Geometry check sheet. Reference: the model listing, model coordinates, mm. A direction names the side the tool comes from. Round coordinates to 2 decimals unless told otherwise and drop trailing zeros. Loops run counter-clockwise (first coordinate to the right, second up) from the corner with the lowest first, then second, coordinate; pieces in that order, holes last. Notation, with made-up numbers: (-28, 75.25) -> (21, 75.25) arc R13 ccw to (21, 85.25) -> close; hole circle Ø11 at (-36.5, -21). An arc over 180 degrees is marked (long way). Use one line per item in the form item = value.
from build123d import *

# Parameters (mm, degrees)
SKETCH1_W           = 34.925
SKETCH1_H           = 34.925
SKETCH1_R           = 1.5
BOSS_EXTRUDE1_DEPTH = 4
CUT_EXTRUDE1_DEPTH  = 5.08
FILLET1_R           = 3
CUT_EXTRUDE2_DEPTH  = 5.08


with BuildPart() as part:
    # Sketch1 → Boss-Extrude1 (new body)
    with BuildSketch(Plane.XY):
        Rectangle(SKETCH1_W, SKETCH1_H)
        with Locations((-12.7, 12.7)):
            Circle(SKETCH1_R, mode=Mode.SUBTRACT)
        with Locations((12.7, 12.7)):
            Circle(SKETCH1_R, mode=Mode.SUBTRACT)
        with Locations((-12.7, -12.7)):
            Circle(SKETCH1_R, mode=Mode.SUBTRACT)
        with Locations((12.7, -12.7)):
            Circle(SKETCH1_R, mode=Mode.SUBTRACT)
        Circle(SKETCH1_R, mode=Mode.SUBTRACT)
    extrude(amount=BOSS_EXTRUDE1_DEPTH)

    # Sketch2 → Cut-Extrude1 (cut)
    with BuildSketch(Plane.XY.offset(4)):
        Polygon((-5.656854249, 0), (-17.4625, 11.805645751), (-17.4625, -11.805645751), align=None)
        Polygon((-11.805645751, 17.4625), (0, 5.656854249), (11.805645751, 17.4625), align=None)
        Polygon((17.4625, 11.805645751), (5.656854249, 0), (17.4625, -11.805645751), align=None)
        Polygon((11.805645751, -17.4625), (0, -5.656854249), (-11.805645751, -17.4625), align=None)
    extrude(amount=-CUT_EXTRUDE1_DEPTH, mode=Mode.SUBTRACT)

    # Fillet1
    fillet1_edges = [part.edges().sort_by_distance(p)[0] for p in [
        (-17.4625, 17.4625, 2),
        (17.4625, 17.4625, 2),
        (17.4625, -17.4625, 2),
        (-17.4625, -17.4625, 2),
        (5.656854249, 0, 2),
        (0, 5.656854249, 2),
        (0, -5.656854249, 2),
        (-5.656854249, 0, 2),
    ]]
    fillet(fillet1_edges, radius=FILLET1_R)

    # Sketch3 → Cut-Extrude2 (cut)
    with BuildSketch(Plane(origin=(0, 0, 0), x_dir=(-1, 0, 0), z_dir=(0, 0, -1))):
        with BuildLine():
            Line((-14.7, -9.043145751), (-3.406944413, -2.095884006))
            ThreePointArc((-3.406944413, -2.095884006), (-4, 0), (-3.406944413, 2.095884006))
            Line((-3.406944413, 2.095884006), (-14.7, 9.043145751))
            Line((-14.7, 9.043145751), (-7.778174593, 2.121320344))
            ThreePointArc((-7.778174593, 2.121320344), (-6.899494937, 0), (-7.778174593, -2.121320344))
            Line((-7.778174593, -2.121320344), (-14.7, -9.043145751))
        make_face()
    extrude(amount=-CUT_EXTRUDE2_DEPTH, mode=Mode.SUBTRACT)


solid = part.part
1. Section check C-C (x = -12.7). Record the boundary of the cut face in (y, z), then the cut area to 3 significant figures.
Return value:
outline = (-17.46, 0) -> (-14.2, 0) -> (-14.2, 4) -> (-17.46, 4) -> close; (-11.2, 0) -> (-7.04, 0) -> (-7.04, 4) -> (-11.2, 4) -> close; (7.04, 0) -> (11.2, 0) -> (11.2, 4) -> (7.04, 4) -> close; (14.2, 0) -> (17.46, 0) -> (17.46, 4) -> (14.2, 4) -> close
area = 59.4 mm2
2. Gauge pin test, flat end, axial feed: pin 1 (1.5 mm diameter, centred on x = 7.5, z = 0.5, fed in from +Y). Record the tip position at first contact, or that the pin passes through.
Return value:
pin_1 = 13.91
3. Section check B-B (z = 1.6). Count the separate pieces of the cut face and the enclosed holes in it, then the cut area to 3 significant figures.
Return value:
separate_pieces = 1
enclosed_holes = 5
area = 583 mm2
4. Mould release check, pull along Y, two halves, no side actions. Record for faces 5 (the cylindrical face through (0, 6.9, 2)), 6 (the cylindrical face through (4, 0, 2)), 7 (the flat face through (-6.896, -12.553, 2.028)), 8 (the cylindrical face through (-1.5, 0.07, 1.97)): released by +Y, released by -Y, zero draft, split by the parting line, or undercut.
Return value:
face_5 = released by +Y
face_6 = undercut
face_7 = released by -Y
face_8 = undercut
5. Section check A-A (y = 0). Record the boundary of the cut face in (x, z).
Return value:
outline = (-6.9, 0) -> (-1.5, 0) -> (-1.5, 4) -> (-6.9, 4) -> close; (1.5, 0) -> (4, 0) -> (4, 4) -> (1.5, 4) -> close
6. Tool access check on faces 1 (the flat face through (9.1, -5.6, 2)), 2 (the flat face through (6.896, 12.553, 2.028)), 3 (the flat face through (7.031, -12.688, 2.028)), 4 (the flat face through (-12.688, -7.031, 2.028)). Record the directions out of +Z, -Z, +X, -X, +Y, -Y that give a thin tool (end or side, any length) a straight path to the whole face; none if there is none.
Return value:
face_1 = +Z, -Z, +X
face_2 = +Z, -Z, +Y
face_3 = +Z, -Z, -Y
face_4 = +Z, -Z, -X
7. Section check D-D (x = 6). Record the boundary of the cut face in (y, z).
Return value:
outline = (-11.66, 0) -> (-3.69, 0) -> (-3.69, 4) -> (-11.66, 4) -> close; (3.69, 0) -> (11.66, 0) -> (11.66, 4) -> (3.69, 4) -> close
8. Material ranges on line 1 along Y through (x, z) = (0, 1.6); line 2 along Y through (x, z) = (-12.7, 0.9); line 3 along Y through (x, z) = (3.5, 3.75), recorded low to high.
Return value:
line_1 = -6.9 to -1.5, 1.5 to 6.9
line_2 = -17.46 to -14.2, -11.2 to -7.04, 7.04 to 11.2, 14.2 to 17.46
line_3 = -9.16 to -2.15, -1.94 to 1.94, 2.15 to 9.16
